Here's how the part is built. I have some questions about the finished solid (model axes, mm). Face numbers are marked on the shaded views. Round coordinates to 2 decimals unless told otherwise and drop trailing zeros. Answer as CSV lines item,"result".
```python
from build123d import *

# Parameters (mm, degrees)
F0_R     = 6.35
F2_W     = 19.05
F2_H     = 19.05
F5_D     = 6.5278
F5_DEPTH = 12.7
F5_TIP   = 1.9611489744


with BuildPart() as f3:
    # F0 (on Top) → F3 section 0
    with BuildSketch(Plane.XY):
        Circle(F0_R)
    # F2 (on offset) → F3 section 1
    with BuildSketch(Plane.XY.offset(25.4)):
        Rectangle(F2_W, F2_H)
    loft()

    # F5
    with Locations(Plane.XY.offset(25.4)):
        with Locations((0, 0)):
            Hole(F5_D / 2, depth=F5_DEPTH)
            with Locations((0, 0, -(F5_DEPTH + F5_TIP / 2))):  # 118° drill point
                Cone(0, F5_D / 2, F5_TIP, mode=Mode.SUBTRACT)


solid = f3.part
```
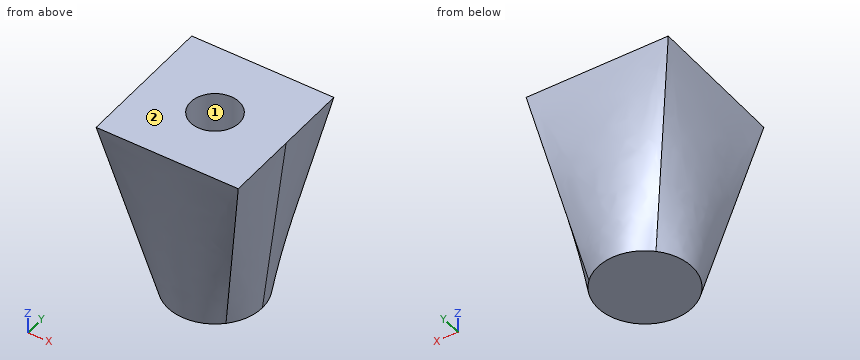
1. For pin 1 Ø5 at (y, z) = (-7.5, 14) entering from -X; pin 2 Ø2 at (y, z) = (-1.5, 16.5) entering from +X; pin 3 Ø6 at (x, y) = (0, 0) entering from +Z, each with a flat end and sliding along its axis, tell me the tip position at first contact or that it passes through.
Numbers:
pin 1,"stops at x = -7.93"
pin 2,"stops at x = 8.52"
pin 3,"stops at z = 12.54"
2. If we mould it in two halves opening along Y, with no side actions, what happens to the marked faces 1 and 2? For each: released by +Y, released by -Y, zero draft, split by the parting line, or undercut.
Numbers:
face 1,"undercut"
face 2,"zero draft"
3. If I drill on line 1 (X direction, y = -0.5, z = 18); line 2 (X direction, y = 3, z = 22.5); line 3 (Y direction, x = 0, z = 20.5), over which ranges is the centre line in solid material (lowest first)?
Numbers:
line 1,"x = -8.6 to -3.23, 3.23 to 8.6"
line 2,"x = -9.14 to -1.29, 1.29 to 9.14"
line 3,"y = -8.91 to -3.26, 3.26 to 8.91"
